Can you work these out from the model? Positions are in its coordinate system, mm. A direction names the side the tool comes from. Round coordinates to 2 decimals unless told otherwise and drop trailing zeros. Order: outer loops, then holes, each group sorted by start corner. A loop starts at its lowest first (then second) coordinate and runs counter-clockwise, first axis right, second up. Notation, with made-up numbers: (-40, 20) - (-35, 20) arc R24 cw to (-35, 42) - close; hole circle Ø4 at (14.5, -15.5). An arc over 180 degrees is marked (long way). Write item = value, one per line.
Autodesk Fusion 360 part; units mm, degrees
sketch "Main" plane through (0, 0, 0) normal (0, 1, 0) x (1, 0, 0)
  line L0 (0, 0) -> (35, 0)
  line L1 (35, 0) -> (35, -21)
  line L2 (-19.4678, -44.3397) -> (-14.4678, -53)
  line L3 (-19.4678, -44.3397) -> (0, -33.1)
  line L4 (0, -33.1) -> (0, 0)
  line L5 (-14.4678, -53) -> (27, -29.0585)
  line L6 (35, -21) -> (27, -21)
  line L7 (27, -21) -> (27, -29.0585)
  dimension "d1" = 35
  dimension "d2" = 21
  dimension "d4" = 10
  dimension "d5" = 60
  dimension "d7" = 53
  dimension "d34" = 33.1
  dimension "d35" = 8
extrude "Extrude1" add sketch "Main" along normal blind 32
sketch "Upper Cut " plane through (19.3327, 0, 33.4853) normal (0.5, 0, 0.866) x (0, 1, 0)
  line L0 (0, 39.0295) -> (0, -8.8534)
  line L1 (32, -8.8534) -> (32, 39.0295)
  line L2 (32, 39.0295) -> (0, 39.0295)
  line L3 (0, -30.3109) -> (32, -30.3109) construction
  line L4 (16, 39.0295) -> (16, -30.3109) construction
  arc A0 (21.8411, 34.4013) -> (10.1589, 34.4013) centre (16, 33.0295) ccw
  line L5 (10.1589, 34.4013) -> (0, -8.8534)
  line L6 (21.8411, 34.4013) -> (32, -8.8534)
  line L7 (0, -8.8534) -> (32, -8.8534)
  dimension "d11" = 6
extrude "Extrude2" cut sketch "Upper Cut " against normal blind 43 contours L0 L2 A0 L5 | L1 L2 A0 L6
sketch "Tube Extension" plane through (19.3327, 0, 33.4853) normal (0.5, 0, 0.866) x (0, 1, 0)
  line L0 (32, -8.8534) -> (21.8411, 34.4013)
  arc A0 (21.8411, 34.4013) -> (10.1589, 34.4013) centre (16, 33.0295) ccw
  line L1 (10.1589, 34.4013) -> (0, -8.8534)
  circle A1 centre (16, 33.0295) radius 6
  line L2 (0, -8.8534) -> (32, -8.8534)
  dimension "d14" = 12
extrude "Extrude3" add sketch "Tube Extension" along normal blind 7 contours A0 A1
sketch "Tube Hole" plane through (22.8327, 0, 39.5474) normal (0.5, 0, 0.866) x (0, 1, 0)
  circle A0 centre (16, 33.0295) radius 6
  circle A1 centre (16, 33.0295) radius 2.1
  dimension "d17" = 4.2
extrude "Extrude4" cut sketch "Tube Hole" against normal up to surface (17 mm away) contours A1
fillet "Fillet1" radius 10 1 edges at (0, 16, 33.1)
sketch "Servo Holes" plane through (19.3327, 0, 33.4853) normal (0.5, 0, 0.866) x (0, 1, 0)
  arc A0 (10.1589, 34.4013) -> (21.8411, 34.4013) centre (16, 33.0295) ccw
  line L0 (10.1589, 34.4013) -> (0, -8.8534)
  line L1 (32, -8.8534) -> (21.8411, 34.4013)
  line L2 (16, 27.0295) -> (16, -8.8534) construction
  line L3 (9.6, 21.4466) -> (22.4, 21.4466)
  line L4 (22.4, 21.4466) -> (22.4, -2.3534)
  line L5 (22.4, -2.3534) -> (9.6, -2.3534)
  line L6 (9.6, -2.3534) -> (9.6, 21.4466)
  circle A1 centre (16, 23.9466) radius 1.8
  circle A2 centre (16, -4.8534) radius 1.8
  line L7 (0, -8.8534) -> (32, -8.8534)
  dimension "d22" = 12.8
  dimension "d23" = 23.8
  dimension "d24" = 6.4
  dimension "d28" = 3.6
  dimension "d29" = 3.6
  dimension "d30" = 28.8
  dimension "d31" = 2.5
  dimension "d36" = 6.5
extrude "Extrude5" cut sketch "Servo Holes" against normal blind 17.5 contours L3 L4 L5 L6
extrude "Extrude6" cut sketch "Servo Holes" against normal blind 4 contours A1 | A2
fillet "Fillet3" radius 2 1 edges at (27, 16, 29.0585)
sketch "Top Plate Holes" plane through (0, 0, 21) normal (0, 0, 1) x (-1, 0, 0)
  line L0 (-27, 0) -> (-35, 0)
  line L1 (-35, 0) -> (-35, -32)
  line L2 (-35, -32) -> (-27, -32)
  line L3 (-27, -32) -> (-27, 0)
  line L4 (-31, -32) -> (-31, 0) construction
  circle A0 centre (-31, -27) radius 2.4
  circle A1 centre (-31, -5) radius 2.4
  dimension "d41" = 4.8
  dimension "d42" = 4.8
  dimension "d44" = 22
  dimension "d45" = 5
extrude "Extrude7" cut sketch "Top Plate Holes" against normal blind 8 contours A0 | A1
sketch "Base Holes" plane through (0, 0, 0) normal (0, 0, -1) x (1, 0, 0)
  line L0 (10.223, 0) -> (0, -2.0793)
  line L1 (0, -2.0793) -> (0, -29.9207)
  line L2 (0, -29.9207) -> (10.223, -32)
  line L3 (10.223, -32) -> (35, -32)
  line L4 (35, -32) -> (35, 0)
  line L5 (35, 0) -> (10.223, 0)
  circle A0 centre (6, -6) radius 2.4
  circle A1 centre (29, -6) radius 2.4
  circle A2 centre (6, -26) radius 2.4
  circle A3 centre (29, -26) radius 2.4
  dimension "d59" = 4.8
  dimension "d61" = 6
  dimension "d62" = 6
  dimension "d65" = 23
  dimension "d66" = -20
extrude "Extrude8" cut sketch "Base Holes" against normal blind 8 contours A0 | A1 | A2 | A3
sketch "Servo Wires " plane through (-18.5733, 0, 10.7233) normal (0.866, 0, -0.5) x (0, 1, 0)
  line L0 (9.6, 28.6269) -> (22.4, 28.6269)
  line L1 (22.4, 28.6269) -> (22.4, 38.6654)
  line L2 (22.4, 38.6654) -> (9.6, 38.6654)
  line L3 (9.6, 38.6654) -> (9.6, 28.6269)
  line L4 (12, 33.6269) -> (20, 33.6269)
  line L5 (20, 33.6269) -> (20, 28.6269)
  line L6 (20, 28.6269) -> (12, 28.6269)
  line L7 (12, 28.6269) -> (12, 33.6269)
  dimension "d93" = 8
  dimension "d94" = 2.4
  dimension "d95" = 5
extrude "Extrude9" cut sketch "Servo Wires " against normal blind 2.3 contours L0 L4 L5 L6 L7
fillet "Fillet4" radius 1.4 3 edges at (-1.7598, 16, 39.8451) (-4.9921, 12, 38.8467) (-4.9921, 20, 38.8467)
(1) If we section it at C-C (y = 6): Write out the boundary of the cut face in (x, z).
Computed:
outline = (-0.99, 31.67) arc R10 cw to (0, 27.33) - (0, 0) - (3.6, 0) - (3.6, 8) - (8.4, 8) - (8.4, 0) - (26.6, 0) - (26.6, 8) - (31.4, 8) - (31.4, 0) - (35, 0) - (35, 21) - (33.18, 21) - (33.18, 13) - (28.82, 13) - (28.82, 21) - (27, 21) - (27, 27.9) arc R2 ccw to (26, 29.64) - (4.88, 41.83) - close
(2) Thinking about a two-plate mould opening in Z: for faces 1 (the face through (0, 16, 11)), 2 (the face through (-1.377, 7.945, 32.39)), 3 (the face through (31, 27, 13)), 4 (the face through (22.082, 17.717, 29.621)), which applies, +Z half, -Z half, draft (parallel to the pull), parting line (faces both ways), or undercut?
Computed:
face_1 = draft
face_2 = -Z half
face_3 = +Z half
face_4 = undercut
(3) Will these pins go through, and if not, where does the flat tip stop? P1, Ø4, axis at x = 31, y = 5, coming from the -Z side; P2, Ø20.5, axis at x = 9, z = 37, coming from the -Y side; P3, Ø5.5, axis at y = 13.5, z = 24.5, coming from the +X side; P4, Ø2, axis at x = 11.5, z = 28, coming from the +Y side.
Computed:
P1 = 0
P2 = 2.19
P3 = 27
P4 = 29.21
(4) If we section it at D-D (x = 6): Write out the boundary of the cut face in (y, z).
Computed:
outline = (0.86, 0) - (3.6, 0) - (3.6, 8) - (8.4, 8) - (8.4, 0) - (23.6, 0) - (23.6, 8) - (28.4, 8) - (28.4, 0) - (31.14, 0) - (26.3, 41.18) - (22.4, 41.18) - (22.4, 20.98) - (9.6, 20.98) - (9.6, 41.18) - (5.7, 41.18) - close
(5) If we section it at A-A (z = 14.5): Write out the boundary of the cut face in (x, y).
Computed:
outline = (0, 3.78) - (18.59, 0) - (35, 0) - (35, 32) - (18.59, 32) - (0, 28.22) - close; hole circle Ø4.8 at (31, 5); hole circle Ø4.8 at (31, 27)
(6) If we section it at B-B (x = 30): Write out the boundary of the cut face in (y, z).
Computed:
outline = (0, 0) - (3.82, 0) - (3.82, 8) - (8.18, 8) - (8.18, 0) - (23.82, 0) - (23.82, 8) - (28.18, 8) - (28.18, 0) - (32, 0) - (32, 21) - (29.18, 21) - (29.18, 13) - (24.82, 13) - (24.82, 21) - (7.18, 21) - (7.18, 13) - (2.82, 13) - (2.82, 21) - (0, 21) - close
(7) On a 3-axis mill with a long thin cutter (end or side, diameter ignored), from which of +Z, -Z, +X, -X, +Y, -Y can I reach the whole of each face in a straight line? I mean faces 5 (the face through (7, 22.4, 31)), 6 (the face through (-1.895, 16.056, 40.409)), 7 (the face through (31.52, 29.343, 17.056)), 8 (the face through (31, 16, 21)). Say none if no direction works.
Computed:
face_5 = none
face_6 = -Z
face_7 = +Z
face_8 = +Z, +X, +Y, -Y
(8) If I drill on line 1 (X direction, y = 26, z = 3.5); line 2 (Y direction, x = 31, z = 16.5); line 3 (Y direction, x = 29, z = 3), over which ranges is the centre line in solid material (lowest first)? Write a range as from..to.
Computed:
line_1 = 0..3.6, 8.4..26.6, 31.4..35
line_2 = 0..2.6, 7.4..24.6, 29.4..32
line_3 = 0..3.6, 8.4..23.6, 28.4..32
